```python
from build123d import *

# Parameters (mm, degrees)
CROQUIS2_R              = 15
SALIENTE_EXTRUIR1_DEPTH = 20
CROQUIS5_R              = 26
CROQUIS4_R              = 19
CORTAR_EXTRUIR1_REACH   = 72
CROQUIS4_7_R            = 10
SALIENTE_EXTRUIR2_REACH = 147
CROQUIS8_W              = 100
CROQUIS8_H              = 20
CROQUIS9_W              = 100
CROQUIS9_H              = 12
SALIENTE_EXTRUIR3_DEPTH = 125
CROQUIS11_W             = 6
CROQUIS11_H             = 50
SALIENTE_EXTRUIR4_DEPTH = 50
CORTAR_EXTRUIR2_DEPTH   = 50
CORTAR_EXTRUIR3_REACH   = 14
CROQUIS13_R             = 15
CORTAR_EXTRUIR4_REACH   = 14
CROQUIS18_W             = 100
CROQUIS18_H             = 25
CROQUIS20_R             = 20
CROQUIS15_R             = 15
CORTAR_EXTRUIR5_REACH   = 197
CROQUIS22_R             = 8


with BuildPart() as part:
    # Croquis2 → Saliente-Extruir1 (new body)
    with BuildSketch(Plane.XY):
        with BuildLine():
            Line((0, 0), (0, 83))
            ThreePointArc((0, 83), (-33, 116), (-66, 83))
            Line((-66, 83), (-66, 0))
            ThreePointArc((-66, 0), (-70.97918472, -12.02081528), (-83, -17))
            Line((-83, -17), (17, -17))
            ThreePointArc((17, -17), (4.97918472, -12.02081528), (0, 0))
        make_face()
        with Locations((-33, 83)):
            Circle(CROQUIS2_R, mode=Mode.SUBTRACT)
    extrude(amount=SALIENTE_EXTRUIR1_DEPTH)

    # Croquis5 → Recubrir2 section 0
    with BuildSketch(Plane(origin=(0, 0, 0), x_dir=(-1, 0, 0), z_dir=(0, 0, -1))):
        with Locations((33, 83)):
            Circle(CROQUIS5_R)
    # Croquis4 → Recubrir2 section 1
    with BuildSketch(Plane.XY.offset(-50)):
        with Locations((-33, 83)):
            Circle(CROQUIS4_R)
    loft()

    # Croquis4_7 → Cortar-Extruir1 (cut, up to next)
    with BuildSketch(Plane.XY.offset(-50), mode=Mode.PRIVATE) as cortar_extruir1_sk1:
        with Locations((-33, 83)):
            Circle(CROQUIS4_7_R)
    cortar_extruir1_tool1 = extrude(cortar_extruir1_sk1.sketch, amount=CORTAR_EXTRUIR1_REACH, mode=Mode.PRIVATE) & part.part
    add(cortar_extruir1_tool1.solids().sort_by_distance((-33, 83, -50))[0], mode=Mode.SUBTRACT)

    # Croquis8 → Saliente-Extruir2 (add, up to next)
    with BuildSketch(Plane(origin=(0, -29, 0), x_dir=(1, 0, 0), z_dir=(0, 1, 0)), mode=Mode.PRIVATE) as saliente_extruir2_sk1:
        with Locations((-33, -10)):
            Rectangle(CROQUIS8_W, CROQUIS8_H)
    saliente_extruir2_tool1 = extrude(saliente_extruir2_sk1.sketch, amount=SALIENTE_EXTRUIR2_REACH, mode=Mode.PRIVATE) - part.part
    add(saliente_extruir2_tool1.solids().sort_by_distance((-33, -29, 10))[0])

    # Croquis9 → Saliente-Extruir3 (add)
    with BuildSketch(Plane.XY.offset(20)):
        with Locations((-33, -23)):
            Rectangle(CROQUIS9_W, CROQUIS9_H)
    extrude(amount=SALIENTE_EXTRUIR3_DEPTH)

    # Croquis11 → Saliente-Extruir4 (add)
    with BuildSketch(Plane.XY.offset(20)):
        with Locations((-33, 8)):
            Rectangle(CROQUIS11_W, CROQUIS11_H)
    extrude(amount=SALIENTE_EXTRUIR4_DEPTH)

    # Croquis12 → Cortar-Extruir2 (cut)
    with BuildSketch(Plane(origin=(-30, 0, 0), x_dir=(0, 0, -1), z_dir=(1, 0, 0))):
        Polygon((-70, -17), (-20, 33), (-70, 33), align=None)
    extrude(amount=-CORTAR_EXTRUIR2_DEPTH, mode=Mode.SUBTRACT)

    # Croquis13 → Cortar-Extruir3 (cut, up to next)
    with BuildSketch(Plane(origin=(0, -17, 0), x_dir=(1, 0, 0), z_dir=(0, 1, 0)), mode=Mode.PRIVATE) as cortar_extruir3_sk1:
        with Locations((-33, -100)):
            Circle(CROQUIS13_R)
    cortar_extruir3_tool1 = extrude(cortar_extruir3_sk1.sketch, amount=-CORTAR_EXTRUIR3_REACH, mode=Mode.PRIVATE) & part.part
    add(cortar_extruir3_tool1.solids().sort_by_distance((-33, -17, 100))[0], mode=Mode.SUBTRACT)

    # Croquis18 → Cortar-Extruir4 (cut, up to next)
    with BuildSketch(Plane(origin=(0, -17, 0), x_dir=(1, 0, 0), z_dir=(0, 1, 0)), mode=Mode.PRIVATE) as cortar_extruir4_sk1:
        with Locations((-33, -132.5)):
            Rectangle(CROQUIS18_W, CROQUIS18_H)
    cortar_extruir4_tool1 = extrude(cortar_extruir4_sk1.sketch, amount=-CORTAR_EXTRUIR4_REACH, mode=Mode.PRIVATE) & part.part
    add(cortar_extruir4_tool1.solids().sort_by_distance((-33, -17, 132.5))[0], mode=Mode.SUBTRACT)

    # Croquis20 → Recubrir6 section 0
    with BuildSketch(Plane.XZ.offset(29)):
        with Locations((-33, 100)):
            Circle(CROQUIS20_R)
    # Croquis15 → Recubrir6 section 1
    with BuildSketch(Plane(origin=(0, -79, 0), x_dir=(1, 0, 0), z_dir=(0, 1, 0))):
        with Locations((-33, -100)):
            Circle(CROQUIS15_R)
    loft()

    # Croquis22 → Cortar-Extruir5 (cut, up to next)
    with BuildSketch(Plane.XZ.offset(79), mode=Mode.PRIVATE) as cortar_extruir5_sk1:
        with Locations((-33, 100)):
            Circle(CROQUIS22_R)
    cortar_extruir5_tool1 = extrude(cortar_extruir5_sk1.sketch, amount=-CORTAR_EXTRUIR5_REACH, mode=Mode.PRIVATE) & part.part
    add(cortar_extruir5_tool1.solids().sort_by_distance((-33, -79, 100))[0], mode=Mode.SUBTRACT)


solid = part.part
```
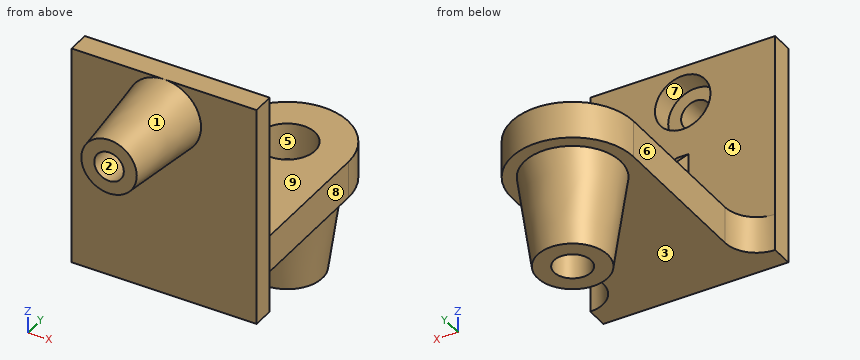
Input: part model. Units: mm. Frame: model coordinates. Face numbers are marked on the shaded views. A direction names the side the tool comes from. Coordinates: 2 decimals unless noted, no trailing zeros. Write each loop counter-clockwise with the first axis right and the second up, starting at its lowest first coordinate (ties: lowest second). Pieces come first, ordered by that corner, then holes. Notation, with made-up numbers: M 12.25,73 L 66.25,73 A11 ccw 66.25,87 Z; hole C 39.25,53 d2. An arc over 180 degrees is marked long. Use one line per item in the form item = value.
Q1. Section B-B (z = -17). Return loops of the section in (x, y), plus the area to 3 significant figures.
Answer below:
outline = C -33,83 d47.24; hole C -33,83 d20
area = 1,440 mm²
Q2. Section C-C (x = 8.5). Return loops of the section in (y, z), plus the area to 3 significant figures.
Answer below:
outline = M -29,0 L -14.72,0 L -14.72,20 L -17,20 L -17,120 L -29,120 Z
area = 1,490 mm²
Q3. Set-up query: the marked faces 5, 6, 7, 8 and 9. Return all of +Z, -Z, +X, -X, +Y, -Y with unobstructed straight access to the full face (end or side cutting, diameter ignored); none if empty.
Answer below:
face_5 = +Z
face_6 = +Z, -Z, -X, +Y
face_7 = +Y
face_8 = +Z, -Z, +X, +Y
face_9 = +Z, +Y
Q4. Section A-A (y = 11). Return loops of the section in (x, z).
Answer below:
outline = M -66,0 L 0,0 L 0,20 L -30,20 L -30,42 L -36,42 L -36,20 L -66,20 Z
Q5. Draft query along Z for the marked faces 1, 2, 3 and 4. Return one class per face: released by +Z, released by -Z, zero draft, split by the parting line, or undercut.
Answer below:
face_1 = split by the parting line
face_2 = undercut
face_3 = released by -Z
face_4 = zero draft
Q6. First-contact query: pin 1 (25 mm diameter, centred on y = -1, z = 41, fed in from -X); pin 2 (12 mm diameter, centred on x = -56.5, z = 29.5, fed in from +Y); pin 3 (1 mm diameter, centred on x = -51.5, y = 26, fed in from -Z). Flat tips, straight axial feed; report the tip coordinate or a pass-through.
Answer below:
pin_1 = -36
pin_2 = -17
pin_3 = 0
Q7. Material intervals for probe 1 along Z at (x, y) = (-33, -25.25); probe 2 along Y at (x, z) = (-33, 6); probe 3 along X at (y, z) = (-20.5, 100), sorted ascending. Write a range as from..to.
Answer below:
probe_1 = 0..85, 115..120
probe_2 = -29..68, 98..116
probe_3 = -83..-48, -18..17
